Input: dimensioned drawing with shaded views. Units: mm. Origin: part minimum x, y, z. A direction names the side the tool comes from. Round coordinates to 2 decimals unless told otherwise and drop trailing zeros. Loops run counter-clockwise (first coordinate to the right, second up) from the corner with the lowest first, then second, coordinate; pieces in that order, holes last. Notation, with made-up numbers: (-32, 8) - (-21, 8) arc R24 ccw to (-21, 36) - close; hole circle Ø10 at (7, -0.75). An arc over 180 degrees is marked (long way). Answer as a JSON object with one key per item and string values. Group by question number.
Item 1: Draft query along Y for the marked faces 1, 2, 3 and 4. Return one class per face: released by +Y, released by -Y, zero draft, split by the parting line, or undercut.
Item 2: First-contact query: pin 1 (6 mm diameter, centred on x = 9.525, y = 8.89, fed in from -Z). Flat tip, straight axial feed; report the tip coordinate or a pass-through.
Item 3: Line query: line 1 (X direction, y = 9, z = 9.75); line 2 (X direction, y = 12, z = 8.89); line 3 (Z direction, x = 20, y = 5.25). Output: solid intervals per line, ascending.
Item 4: Section A-A (y = 8.89). Count the separate pieces of the cut face and the enclosed holes in it, plus the area to 3 significant figures.
Item 5: Section C-C (x = 10). Return the cut outline in (y, z).
Item 6: Reachability of the marked faces 5 and 6 from +Z, -Z, +X, -X, +Y, -Y: full face, straight path, thin tool, end or side. Return the list, or none.
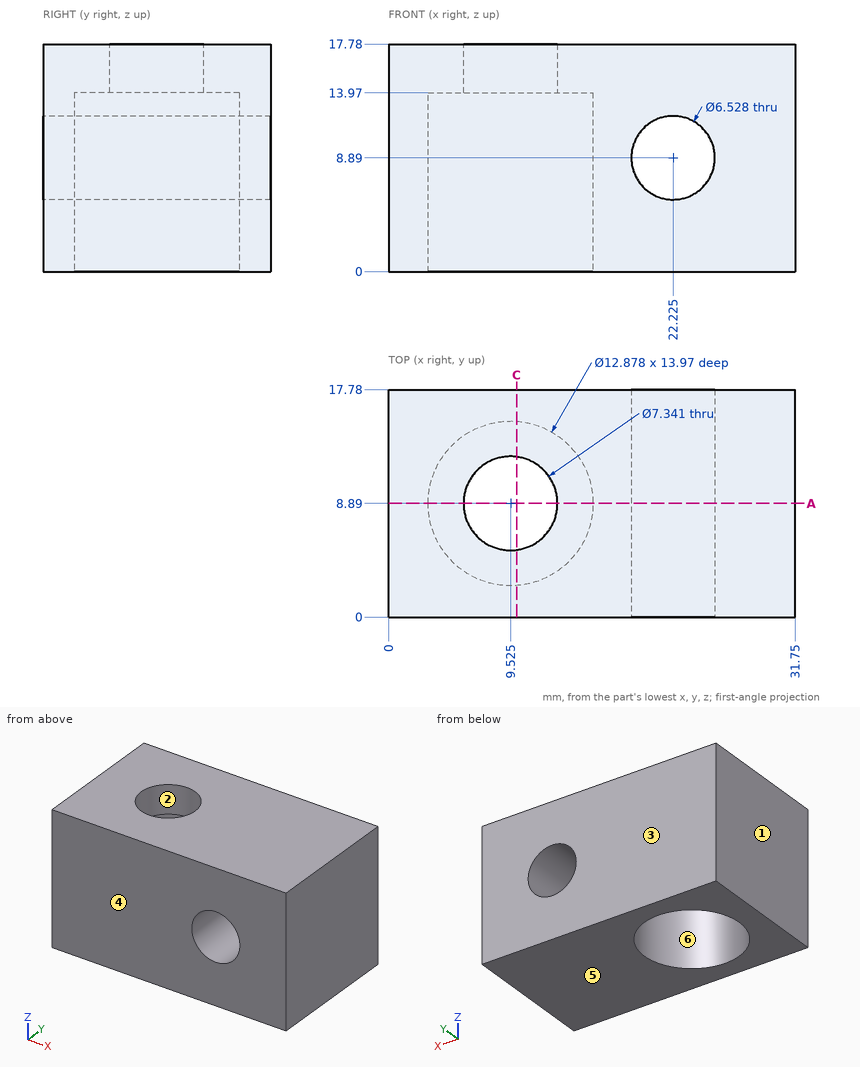
Values:
{
 "1": {"face 1": "zero draft", "face 2": "undercut", "face 3": "released by +Y", "face 4": "released by -Y"},
 "2": {"pin 1": "passes through"},
 "3": {"line 1": "x = 0 to 3.09, 15.96 to 19.08, 25.37 to 31.75", "line 2": "x = 0 to 3.89, 15.16 to 18.96, 25.49 to 31.75", "line 3": "z = 0 to 6.5, 11.28 to 17.78"},
 "4": {"separate pieces": "2", "enclosed holes": "1", "area": "323 mm^2"},
 "5": {"outline": "(0, 0) - (2.47, 0) - (2.47, 13.97) - (5.25, 13.97) - (5.25, 17.78) - (0, 17.78) - close; (12.53, 13.97) - (15.31, 13.97) - (15.31, 0) - (17.78, 0) - (17.78, 17.78) - (12.53, 17.78) - close"},
 "6": {"face 5": "-Z, +X, -X, +Y, -Y", "face 6": "-Z"}
}
